```python
from build123d import *

# Parameters (mm, degrees)
SKETCH_1_R                        = 60
EXTRUDE_1_DEPTH                   = 26.5
SKETCH_2_R                        = 26
EXTRUDE_2_DEPTH                   = 60
CUT_EXTRUDE_START                 = -14
SKETCH_3_R                        = 55.5
SKETCH_3_R_2                      = 26
CUT_EXTRUDE_1_DEPTH               = 14
CUT_EXTRUDE_2_DEPTH               = 104.923048454
CUT_EXTRUDE_START_2               = -16
SKETCH_5_R                        = 26
SKETCH_5_R_2                      = 24
CUT_EXTRUDE_3_DEPTH               = 3
HOLE_WIZARD_12_0_12_1_D           = 12
HOLE_WIZARD_12_0_12_1_CSINK_D     = 12.05
HOLE_WIZARD_12_0_12_1_CSINK_ANGLE = 90
CHAMFER_1_SIZE                    = 1
FILLET_1_R                        = 2


# Read off the part's stored shape, not the designer's step: M8 螺纹孔的螺纹孔钻头1
with BuildPart() as part:
    # 草图1 → 凸台-拉伸1 (new body)
    with BuildSketch(Plane.XY):
        Circle(SKETCH_1_R)
    extrude(amount=EXTRUDE_1_DEPTH)

    # 草图2 → 凸台-拉伸2 (add)
    with BuildSketch(Plane.XY):
        Circle(SKETCH_2_R)
    extrude(amount=EXTRUDE_2_DEPTH)

    # 草图3 → 切除-拉伸1 (cut)
    with BuildSketch(Plane.XY.offset(26.5).offset(CUT_EXTRUDE_START)):
        Circle(SKETCH_3_R)
        Circle(SKETCH_3_R_2, mode=Mode.SUBTRACT)
    extrude(amount=CUT_EXTRUDE_1_DEPTH, mode=Mode.SUBTRACT)

    # 草图4 → 切除-拉伸2 (cut, through all)
    with BuildSketch(Plane.XY.offset(60)):
        with BuildLine():
            Line((-4, 12.369316877), (-4, 16))
            Line((-4, 16), (4, 16))
            Line((4, 16), (4, 12.369316877))
            ThreePointArc((4, 12.369316877), (0, -13), (-4, 12.369316877))
        make_face()
    extrude(amount=-CUT_EXTRUDE_2_DEPTH, mode=Mode.SUBTRACT)

    # M8 螺纹孔的螺纹孔钻头1 outline → M8 螺纹孔的螺纹孔钻头1 (revolve, cut)
    with BuildSketch(Plane.XY.offset(45.5)):
        Polygon((0, -26.000014008), (3.425014008, -26.000014008), (3.399999801, -25.974999801), (3.4, -12.54744384), (0, -12.54744384), align=None)
    revolve(axis=Axis((0, 0, 45.5), (0, 1, 0)), mode=Mode.SUBTRACT)

    # 草图5 → 切除-拉伸3 (cut)
    with BuildSketch(Plane.XY.offset(60).offset(CUT_EXTRUDE_START_2)):
        with Locations(Location((0, 0, 0), (0, 0, 263.260542122))):
            Circle(SKETCH_5_R)
        Circle(SKETCH_5_R_2, mode=Mode.SUBTRACT)
    extrude(amount=CUT_EXTRUDE_3_DEPTH, mode=Mode.SUBTRACT)

    # Ø12.0 (12) 直径孔1 (through all)
    with Locations(Plane.XY.offset(12.5)):
        with Locations((21, 36.373066959), (42, 0), (21, -36.373066959), (-21, -36.373066959), (-42, 0), (-21, 36.373066959)):
            CounterSinkHole(HOLE_WIZARD_12_0_12_1_D / 2, HOLE_WIZARD_12_0_12_1_CSINK_D / 2, counter_sink_angle=HOLE_WIZARD_12_0_12_1_CSINK_ANGLE)

    # 倒角1
    chamfer_1_edges = [part.edges().sort_by_distance(p)[0] for p in [
        (-60, 0, 26.5),
    ]]
    chamfer(chamfer_1_edges, length=CHAMFER_1_SIZE)

    # 圆角1
    fillet_1_edges = [part.edges().sort_by_distance(p)[0] for p in [
        (-55.5, 0, 12.5),
    ]]
    fillet(fillet_1_edges, radius=FILLET_1_R)


solid = part.part
```
Design review of the part built by this model. Coordinates are the model's own, in mm. A direction names the side the tool comes from. Coordinates: 2 decimals unless noted, no trailing zeros. Loops run counter-clockwise (first coordinate to the right, second up) from the corner with the lowest first, then second, coordinate; pieces in that order, holes last. Notation, with made-up numbers: (83.25, -31.75) - (118.25, -31.75) arc R18 cw to (118.25, -26.75) - close; hole circle Ø4 at (-33, -18). An arc over 180 degrees is marked (long way). Use CSV: the item, a comma, the result in double quotes. Start each with the question number.
1) Wall thickness on L1, parallel to X at y = 0, z = 52; L2, parallel to Y at x = 21, z = 9; L3, parallel to Y at x = 0, z = 35: over which ranges is each line inside the solid? List them lowest first. Write a range as from..to.
2) The part is to be moulded in two halves that separate along X. For faces 4 (the flat face through (-4, 14, 30)), 5 (the flat face through (-14, 1, 0)), 6 (the cylindrical face through (22.301, 30.516, 6.15)), 7 (the cylindrical face through (1.01, 23.98, 45.48)), say which applies: +X half, -X half, draft (parallel to the pull), parting line (faces both ways), or undercut.
3) Consider section B-B on x = 20. Give the number of separate pieces and of enclosed holes in the cut face, then the cut area to 3 significant figures.
4) Tool access review of faces 1 (the flat face through (39, 40, 26.5)), 2 (the cylindrical face through (48, 0, 6)), 3 (the cylindrical face through (-3.4, -19.2, 45.4)): name each direction out of +Z, -Z, +X, -X, +Y, -Y from which nothing blocks a thin tool from reaching the whole face with its end or side.
5) Consider section A-A on z = 39. Write out the cut boundary in (x, y), then the cut area to 3 significant figures.
6) For pin 1 Ø14 at (x, y) = (21, 36.37) entering from +Z; pin 2 Ø1.1 at (y, z) = (14, 33) entering from +X; pin 3 Ø4 at (x, z) = (0, 22.5) entering from -Y, all flat-tipped, find the tip position at first contact; note any pin that passes through.
Geometry says:
1,L1,"-26..-13, 13..26"
1,L2,"-56.2..-42.37, -30.37..30.37, 42.37..56.2"
1,L3,"-26..-13, 16..26"
2,face 4,"undercut"
2,face 5,"draft"
2,face 6,"undercut"
2,face 7,"parting line"
3,separate pieces,"3"
3,enclosed holes,"0"
3,area,"2,810 mm^2"
4,face 1,"+Z"
4,face 2,"+Z, -Z"
4,face 3,"-Y"
5,outline,"circle Ø52 at (0, 0); hole (-4, 12.37) arc R13 ccw (long way) to (4, 12.37) - (4, 16) - (-4, 16) - close"
5,area,"1,570 mm^2"
6,pin 1,"z = 12.5"
6,pin 2,"x = 22.25"
6,pin 3,"y = -60"
